Read the model definition and answer for the solid it produces. Units are mm, in the model's axes. Coordinates: 2 decimals unless noted, no trailing zeros. Order: outer loops, then holes, each group sorted by start corner. A loop starts at its lowest first (then second) coordinate and runs counter-clockwise, first axis right, second up. Notation, with made-up numbers: (-24, -18.5) -> (-16, -18.5) arc R12 ccw to (-16, -3.5) -> close; hole circle Ø9 at (33, 4). An arc over 180 degrees is marked (long way). Use CSV: the item, a comma, the result in double quotes.
```python
from build123d import *

# Parameters (mm, degrees)
F0_W     = 28
F0_H     = 28
F1_DEPTH = 500
F2_W     = 32
F2_H     = 32
F2_W_2   = 28
F2_H_2   = 28
F3_DEPTH = 420.3
F4_W     = 100
F4_H     = 100
F5_DEPTH = 6
F6_R     = 41
F7_DEPTH = 25


with BuildPart() as f1:
    # F0 (on Right) → F1 (new body, symmetric)
    with BuildSketch(Plane.YZ):
        with BuildLine():
            ThreePointArc((-450, -14), (-449.414214, -15.414214), (-448, -16))
            Line((-448, -16), (-420, -16))
            ThreePointArc((-420, -16), (-418.585786, -15.414214), (-418, -14))
            Line((-418, -14), (-418, 14))
            ThreePointArc((-418, 14), (-418.585786, 15.414214), (-420, 16))
            Line((-420, 16), (-448, 16))
            ThreePointArc((-448, 16), (-449.414214, 15.414214), (-450, 14))
            Line((-450, 14), (-450, -14))
        make_face()
        with Locations((-434, 0)):
            Rectangle(F0_W, F0_H, mode=Mode.SUBTRACT)
        with BuildLine():
            ThreePointArc((450, 14), (449.414214, 15.414214), (448, 16))
            Line((448, 16), (420, 16))
            ThreePointArc((420, 16), (418.585786, 15.414214), (418, 14))
            Line((418, 14), (418, -14))
            ThreePointArc((418, -14), (418.585786, -15.414214), (420, -16))
            Line((420, -16), (448, -16))
            ThreePointArc((448, -16), (449.414214, -15.414214), (450, -14))
            Line((450, -14), (450, 14))
        make_face()
        with Locations((434, 0)):
            Rectangle(F0_W, F0_H, mode=Mode.SUBTRACT)
    extrude(amount=F1_DEPTH, both=True)

    # F2 (on Front) → F3 (join, symmetric)
    with BuildSketch(Plane.XZ):
        with Locations((-66, -0.042497)):
            Rectangle(F2_W, F2_H)
        with Locations((-66, -0.042497)):
            Rectangle(F2_W_2, F2_H_2, mode=Mode.SUBTRACT)
        with Locations((66, -0.042497)):
            Rectangle(F2_W, F2_H)
        with Locations((66, -0.042497)):
            Rectangle(F2_W_2, F2_H_2, mode=Mode.SUBTRACT)
    extrude(amount=F3_DEPTH, both=True)

    # F4 (on face) → F5 (join)
    with BuildSketch(Plane.XY.offset(15.957503)):
        Rectangle(F4_W, F4_H)
    extrude(amount=-F5_DEPTH)

    # F6 (on face) → F7 (cut)
    with BuildSketch(Plane.XY.offset(15.957503)):
        Circle(F6_R)
    extrude(amount=-F7_DEPTH, mode=Mode.SUBTRACT)


solid = f1.part
```
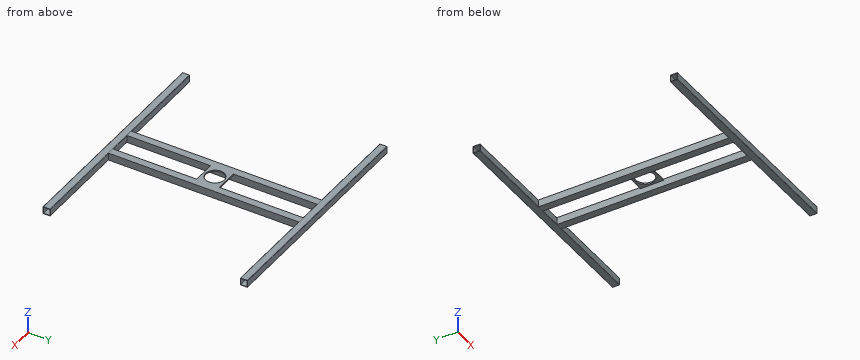
Item 1: Straight lines are drawn through the part: line 1 along Y through (x, z) = (0, 12.5); line 2 along Y through (x, z) = (116.5, -1.5); line 3 along X through (y, z) = (223, 7). For each, find the intervals that lie inside material, in ascending order.
Return value:
line 1,"y = -450 to -448, -420 to -418, -50 to -41, 41 to 50, 418 to 420, 448 to 450"
line 2,"y = -450 to -448, -420 to -418, 418 to 420, 448 to 450"
line 3,"x = -82 to -80, -52 to -50, 50 to 52, 80 to 82"
Item 2: Find section B-B, the plane x = 0. Give the number of separate pieces and of enclosed holes in the cut face, then the cut area to 3 significant figures.
Return value:
separate pieces,"4"
enclosed holes,"2"
area,"581 mm^2"
Item 3: Each of these flat-tipped pins is pushed along its axis until it touches: P1, Ø6, axis at x = 87.5, y = 47.5, coming from the +Z side; P2, Ø14, axis at x = -99, y = 431.5, coming from the -Z side. Where does it stop, or does it pass through?
Return value:
P1,"passes through"
P2,"stops at z = -16"
Item 4: Find section A-A, the plane y = 249. Give the vertices of the cut face in (x, z).
Return value:
outline,"(-82, -16.04) -> (-50, -16.04) -> (-50, 15.96) -> (-82, 15.96) -> close; (50, -16.04) -> (82, -16.04) -> (82, 15.96) -> (50, 15.96) -> close; hole (-80, -14.04) -> (-52, -14.04) -> (-52, 13.96) -> (-80, 13.96) -> close; hole (52, -14.04) -> (80, -14.04) -> (80, 13.96) -> (52, 13.96) -> close"
Item 5: Find section C-C, the plane x = 370. Give the vertices of the cut face in (y, z).
Return value:
outline,"(-450, -14) arc R2 ccw to (-448, -16) -> (-420, -16) arc R2 ccw to (-418, -14) -> (-418, 14) arc R2 ccw to (-420, 16) -> (-448, 16) arc R2 ccw to (-450, 14) -> close; (418, -14) arc R2 ccw to (420, -16) -> (448, -16) arc R2 ccw to (450, -14) -> (450, 14) arc R2 ccw to (448, 16) -> (420, 16) arc R2 ccw to (418, 14) -> close; hole (-448, -14) -> (-420, -14) -> (-420, 14) -> (-448, 14) -> close; hole (420, -14) -> (448, -14) -> (448, 14) -> (420, 14) -> close"
